Input: part model. Units: mm. Frame: model coordinates. A direction names the side the tool comes from. Coordinates: 2 decimals unless noted, no trailing zeros. Loops run counter-clockwise (first coordinate to the right, second up) from the corner with the lowest first, then second, coordinate; pieces in that order, holes last. Notation, with made-up numbers: M 47.25,73.25 L 73.25,73.25 A15 cw 73.25,89.25 Z; hole C 66.25,0 d5. An arc over 180 degrees is marked long. Use a Markdown table: item, result. Add a question column.
1. Section A-A on y = 12.5. Output: boundary loops of the cut face in (x, z).
2. Section B-B on x = -19.8. Output: boundary loops of the cut face in (y, z), then the cut area to 3 significant figures.
3. Line query: L1, parallel to Y at x = -3, z = 2.25; L2, parallel to X at y = 12.5, z = 1.9; L3, parallel to X at y = -12, z = 2.5. Output: solid intervals per line, ascending. Write a range as [from, to].
4. Section C-C on y = 0. Output: boundary loops of the cut face in (x, z).
5. Section D-D on z = 5.5. State how many separate pieces and enclosed holes the cut face has, then the cut area to 3 significant figures.
6. Set-up query: faces 4 (the cylindrical face through (9.6, 12.6, 4.8)), 5 (the flat face through (0, 34.413, 3)), 6 (the cylindrical face through (-29.61, -7.37, 3.24)), 7 (the cylindrical face through (20.39, -7.37, 3.24)), 8 (the cylindrical face through (29.61, -22.37, 3.24)). Return all of +Z, -Z, +X, -X, +Y, -Y with unobstructed straight access to the full face (end or side cutting, diameter ignored); none if empty.
7. Draft query along X for faces 1 (the flat face through (-12.5, -31, 3)), 2 (the cylindrical face through (29.63, 22.32, 3.24)), 3 (the cylindrical face through (9.6, -12.4, 4.8)). Return one class per face: +X half, -X half, draft (parallel to the pull), parting line (faces both ways), or undercut.
8. Pin query (flat end, axial travel): pin 1 (3 mm diameter, centred on x = -12.5, y = 12.5, fed in from +Z); pin 2 (3 mm diameter, centred on y = -16.5, z = 3.5, fed in from -X); pin 3 (1.5 mm diameter, centred on x = -12, z = 2, fed in from +Y); pin 4 (1.4 mm diameter, centred on y = 33, z = 3, fed in from +X). Return the tip coordinate at first contact, or that it passes through.
```python
from build123d import *

# Parameters (mm, degrees)
F0_R     = 1.6
F0_W     = 11.2785340156
F0_H     = 2.8266120087
F0_R_2   = 2.65
F0_R_3   = 4.2
F1_DEPTH = 6.4
F2_R     = 5
F3_R     = 2.9
F4_DEPTH = 3.2


# Not quite as in the source:
# - a feature names something its author has since deleted; it is built from what else it names


with BuildPart() as f1:
    # F0 (on Top) → F1 (new body)
    with BuildSketch(Plane.XY):
        Polygon((-12.5, -40), (12.5, -40), (30, -22.5), (30, -17.5), (20, -7.5), (20, 7.5), (30, 17.5), (30, 22.5), (12.5, 40), (-12.5, 40), (-12.5, 25), (-30, 7.5), (-30, -7.5), (-12.5, -25), align=None)
        with Locations((-12.5, -12.5)):
            Circle(F0_R, mode=Mode.SUBTRACT)
        with Locations((0, -33)):
            Rectangle(F0_W, F0_H, mode=Mode.SUBTRACT)
        with Locations((12.5, -12.5)):
            Circle(F0_R, mode=Mode.SUBTRACT)
        with Locations((20, -20)):
            Circle(F0_R_2, mode=Mode.SUBTRACT)
        with Locations((-19.8, 0)):
            Circle(F0_R_3, mode=Mode.SUBTRACT)
        with Locations((-12.5, 12.5)):
            Circle(F0_R, mode=Mode.SUBTRACT)
        with Locations((12.5, 12.5)):
            Circle(F0_R, mode=Mode.SUBTRACT)
        with Locations((0, 33)):
            Rectangle(F0_W, F0_H, mode=Mode.SUBTRACT)
        with Locations((20, 20)):
            Circle(F0_R_2, mode=Mode.SUBTRACT)
    extrude(amount=F1_DEPTH)

    # F2
    f2_edges = [f1.edges().sort_by_distance(p)[0] for p in [
        (30, 17.5, 3.2),
        (30, 22.5, 3.2),
        (-12.5, -25, 3.2),
        (-12.5, 25, 3.2),
        (-12.5, -40, 3.2),
        (12.5, -40, 3.2),
        (30, -22.5, 3.2),
        (30, -17.5, 3.2),
        (20, -7.5, 3.2),
        (20, 7.5, 3.2),
        (12.5, 40, 3.2),
        (-12.5, 40, 3.2),
        (-30, 7.5, 3.2),
        (-30, -7.5, 3.2),
    ]]
    fillet(f2_edges, radius=F2_R)

    # F3 (on face) → F4 (cut)
    with BuildSketch(Plane.XY.offset(6.4)):
        with Locations((-12.5, 12.5)):
            Circle(F3_R)
        with Locations((12.5, 12.5)):
            Circle(F3_R)
        with Locations((12.5, -12.5)):
            Circle(F3_R)
        with Locations((-12.5, -12.5)):
            Circle(F3_R)
    extrude(amount=-F4_DEPTH, mode=Mode.SUBTRACT)


solid = f1.part
```
Answers below:
| question | item | result |
|---|---|---|
| 1 | outline | M -25,0 L -14.1,0 L -14.1,3.2 L -15.4,3.2 L -15.4,6.4 L -25,6.4 Z; M -10.9,0 L 10.9,0 L 10.9,3.2 L 9.6,3.2 L 9.6,6.4 L -9.6,6.4 L -9.6,3.2 L -10.9,3.2 Z; M 14.1,0 L 25,0 L 25,6.4 L 15.4,6.4 L 15.4,3.2 L 14.1,3.2 Z |
| 2 | outline | M -17.7,0 L -4.2,0 L -4.2,6.4 L -17.7,6.4 Z; M 4.2,0 L 17.7,0 L 17.7,6.4 L 4.2,6.4 Z |
| 2 | area | 173 mm² |
| 3 | L1 | y = [-40, -34.41], [-31.59, 31.59], [34.41, 40] |
| 3 | L2 | x = [-25, -14.1], [-10.9, 10.9], [14.1, 25] |
| 3 | L3 | x = [-25.5, -14.02], [-10.98, 10.98], [14.02, 24.5] |
| 4 | outline | M -30,0 L -24,0 L -24,6.4 L -30,6.4 Z; M -15.6,0 L 20,0 L 20,6.4 L -15.6,6.4 Z |
| 5 | separate pieces | 1 |
| 5 | enclosed holes | 9 |
| 5 | area | 3,130 mm² |
| 6 | face 4 | +Z |
| 6 | face 5 | +Z, -Z |
| 6 | face 6 | +Z, -Z, -X, -Y |
| 6 | face 7 | +Z, -Z, +X |
| 6 | face 8 | +Z, -Z, +X, -Y |
| 7 | face 1 | -X half |
| 7 | face 2 | +X half |
| 7 | face 3 | undercut |
| 8 | pin 1 | passes through |
| 8 | pin 2 | stops at x = -22.5 |
| 8 | pin 3 | stops at y = 38.31 |
| 8 | pin 4 | stops at x = 20.2 |
